Autodesk Inventor part; units mm, degrees
ref_plane "YZ Plane" through (0, 0, 0) normal (1, 0, 0) x (0, 1, 0)
ref_plane "XZ Plane" through (0, 0, 0) normal (0, 1, 0) x (-1, 0, 0)
ref_plane "XY Plane" through (0, 0, 0) normal (0, 0, 1) x (1, 0, 0)
sketch "スケッチ1" plane through (0, 0, 0) normal (0, 1, 0) x (-1, 0, 0)
  circle A0 centre (0, 0) radius 20.5
  dimension "d0" = 41
extrude "押し出し1" add sketch "スケッチ1" along normal blind 23.5
sketch "スケッチ2" plane through (0, 23.5, 0) normal (0, 1, 0) x (1, 0, 0)
  line L0 (0, 0) -> (7, 0)
  circle A0 centre (7, 0) radius 6
  dimension "d3" = 7
  dimension "d4" = 12
extrude "押し出し2" add sketch "スケッチ2" along normal blind 6
sketch "スケッチ3" plane through (7, 29.5, 0) normal (0, 1, 0) x (1, 0, 0)
  circle A0 centre (0, 0) radius 3
  point P0 (-7, 0)
  dimension "d7" = 6
extrude "押し出し3" add sketch "スケッチ3" along normal blind 15
sketch "スケッチ6" plane through (0, 23.5, 0) normal (0, 1, 0) x (1, 0, 0)
  circle A0 centre (0, 0) radius 15.5
  line L0 (0, 0) -> (23.5113, 0) construction
  line L1 (0, 0) -> (25.2681, -14.5885)
  line L2 (0, 0) -> (29.1771, 0) construction
  line L3 (0, 0) -> (-23.275, -13.4378)
  line L4 (0, 0) -> (26.8756, 0) construction
  point P0 (0, 15.5)
  point P1 (-13.4234, -7.75)
  point P2 (13.4234, -7.75)
  dimension "d31" = 31
  dimension "d33" = 30
  dimension "d34" = 150
hole "穴3" at (0, 23.5, -15.5) at (-13.4234, 23.5, 7.75) at (13.4234, 23.5, 7.75) direction (0, -1, 0) diameter 3 depth 10 tip angle 118
sketch "スケッチ7" plane through (0, 0, 0) normal (0, -1, 0) x (1, 0, 0)
  circle A0 centre (0, 0) radius 13.75
  dimension "d42" = 27.5
extrude "押し出し4" add sketch "スケッチ7" along normal blind 38
sketch "スケッチ8" plane through (7, 44.5, 0) normal (0, 1, 0) x (1, 0, 0)
  line L0 (-2.5, 0) -> (-2.5, 1.6583)
  circle A0 centre (0, 0) radius 3
  line L1 (-2.5, 0) -> (-2.5, -1.6583)
  arc A1 (-2.5, 1.6583) -> (-2.5, -1.6583) centre (0, 0) ccw
  point P0 (-7, 0)
extrude "押し出し5" cut sketch "スケッチ8" against normal blind 7.5 contours L1 A0 L0 picked at (-2.6056, -0.897)
fillet "フィレット2" radius 0.5 1 edges at (7.866, 44.5, 2.8723)
properties part number "tamiya"
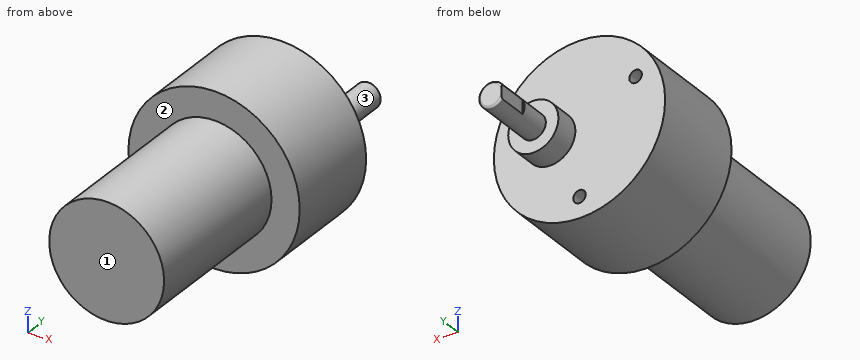
Build history of the part. All positions in model axes, mm. Face numbers are marked on the shaded views. A direction names the side the tool comes from. Round coordinates to 2 decimals unless told otherwise and drop trailing zeros. Write each loop counter-clockwise with the first axis right and the second up, starting at its lowest first coordinate (ties: lowest second). Pieces come first, ordered by that corner, then holes. Notation, with made-up numbers: (46.5, 25) -> (93.5, 25) arc R4 cw to (93.5, 29) -> close; hole circle Ø11 at (81, 28.25). An arc over 180 degrees is marked (long way). Use one line per item in the form item = value.
Q1. Band-saw the part on C-C, the plane y = -28. Write the cut outline in (x, z).
Conclusion:
outline = circle Ø27.5 at (0, 0)
Q2. Drop flat-ended pins along their axis: P1, Ø2.5, axis at x = 0, z = -15.5, coming from the -Y side; P2, Ø8, axis at y = 6.5, z = 11, coming from the +X side; P3, Ø1, axis at x = 15, y = 6, coming from the -Z side. Give the stop position or say it passes through.
Conclusion:
P1 = 0
P2 = 19.27
P3 = -14.49
Q3. Band-saw the part on B-B, the plane z = 12. Write the cut outline in (x, y), then the cut area to 3 significant figures.
Conclusion:
outline = (-16.62, 0) -> (-6.71, 0) -> (-6.71, -38) -> (6.71, -38) -> (6.71, 0) -> (16.62, 0) -> (16.62, 23.5) -> (-16.62, 23.5) -> close
area = 1,290 mm²
Q4. Band-saw the part on D-D, the plane y = 22. Write the cut outline in (x, z), then the cut area to 3 significant figures.
Conclusion:
outline = circle Ø41 at (0, 0); hole circle Ø3 at (-13.42, 7.75); hole circle Ø3 at (0, -15.5); hole circle Ø3 at (13.42, 7.75)
area = 1,300 mm²
Q5. Tool access for the marked faces 1, 2 and 3: list every direction of +Z, -Z, +X, -X, +Y, -Y with a clear straight run to the whole face (end or side of a thin tool).
Conclusion:
face_1 = +Z, -Z, +X, -X, -Y
face_2 = -Y
face_3 = +Y
Q6. Drill centre lines: L1, parallel to Y at x = -10.5, z = 5; L2, parallel to Y at x = 12, z = 13; L3, parallel to X at y = 18, z = 7. Where is each one in solid material? Low to high.
Conclusion:
L1 = -38 to 23.5
L2 = 0 to 23.5
L3 = -19.27 to -14.72, -12.12 to 12.12, 14.72 to 19.27
Q7. Band-saw the part on A-A, the plane x = -8. Write the cut outline in (y, z), then the cut area to 3 significant figures.
Conclusion:
outline = (-38, -11.18) -> (0, -11.18) -> (0, -18.87) -> (23.5, -18.87) -> (23.5, 18.87) -> (0, 18.87) -> (0, 11.18) -> (-38, 11.18) -> close
area = 1,740 mm²
